```python
from build123d import *

# Parameters (mm, degrees)
SKETCH2_W               = 79.756
SKETCH2_H               = 39.795093556
BOSS_EXTRUDE1_DEPTH     = 39.878
SKETCH4_R               = 19.05
CUT_EXTRUDE2_DEPTH      = 1
CUT_EXTRUDE2_DEPTH_BACK = 40.795093555


with BuildPart() as part:
    # Sketch2 → Boss-Extrude1 (new body)
    with BuildSketch(Plane.XY):
        Rectangle(SKETCH2_W, SKETCH2_H)
    extrude(amount=-BOSS_EXTRUDE1_DEPTH)

    # Sketch4 → Cut-Extrude2 (cut, two sides)
    with BuildSketch(Plane(origin=(0, 19.897546778, 0), x_dir=(1, 0, 0), z_dir=(0, 1, 0))) as cut_extrude2_sk:
        Circle(SKETCH4_R)
    extrude(amount=CUT_EXTRUDE2_DEPTH, mode=Mode.SUBTRACT)
    extrude(cut_extrude2_sk.sketch, amount=-CUT_EXTRUDE2_DEPTH_BACK, mode=Mode.SUBTRACT)


solid = part.part
```
For this review, take the finished solid that the model builds, in its own axes (mm). Round coordinates to 2 decimals unless told otherwise and drop trailing zeros. Order: outer loops, then holes, each group sorted by start corner. A loop starts at its lowest first (then second) coordinate and runs counter-clockwise, first axis right, second up.
Q1. Wall thickness on line 1 (X direction, y = -7.5, z = -8.5); line 2 (X direction, y = -14.5, z = -5.5); line 3 (Z direction, x = -0.5, y = -13): over which ranges is each line inside the solid? List them lowest first.
Findings below:
line 1: x = -39.88 to -17.05, 17.05 to 39.88
line 2: x = -39.88 to -18.24, 18.24 to 39.88
line 3: z = -39.88 to -19.04
Q2. We need section A-A, the plane z = -13. Give the boundary of the cut face in (x, y).
Findings below:
outline: (-39.88, -19.9) - (-13.92, -19.9) - (-13.92, 19.9) - (-39.88, 19.9) - close; (13.92, -19.9) - (39.88, -19.9) - (39.88, 19.9) - (13.92, 19.9) - close
Q3. We need section B-B, the plane y = 5. Give the boundary of the cut face in (x, z), plus the area to 3 significant figures.
Findings below:
outline: (-39.88, -39.88) - (39.88, -39.88) - (39.88, 0) - (19.05, 0) arc R19.05 cw to (-19.05, 0) - (-39.88, 0) - close
area: 2,610 mm2
Q4. We need section C-C, the plane x = 0. Give the boundary of the cut face in (y, z), plus the area to 3 significant figures.
Findings below:
outline: (-19.9, -39.88) - (19.9, -39.88) - (19.9, -19.05) - (-19.9, -19.05) - close
area: 829 mm2
Q5. We need section D-D, the plane x = -12.5. Give the boundary of the cut face in (y, z), plus the area to 3 significant figures.
Findings below:
outline: (-19.9, -39.88) - (19.9, -39.88) - (19.9, -14.38) - (-19.9, -14.38) - close
area: 1,010 mm2
Q6. Insertion check: P1, Ø12, axis at x = 1.5, y = -5, coming from the +Z side. The pin has a flat end and moves straight along its axis. Give the tip position at first contact, or say it passes through.
Findings below:
P1: stops at z = -17.51
Q7. Mouldability with a two-part tool opening along X and no side actions: class faces 1 (the flat face through (-1, -19.898, -24)), 2 (the flat face through (-39.878, 0, -20)), 3 (the cylindrical face through (0.419, 0.279, -19.045)) as pulls with the +X half, pulls with the -X half, needs draft (parallel to the pull), parting line crosses it, or undercut.
Findings below:
face 1: needs draft
face 2: pulls with the -X half
face 3: undercut
